Input: part model. Units: mm. Frame: model coordinates. A direction names the side the tool comes from. Round coordinates to 2 decimals unless told otherwise and drop trailing zeros. Loops run counter-clockwise (first coordinate to the right, second up) from the corner with the lowest first, then second, coordinate; pieces in that order, holes last.
1) Section B-B, the plane x = 12. Return loops of the section in (y, z).
2) First-contact query: pin 1 (0.8 mm diameter, centred on x = -17.5, y = 1, fed in from +Z); pin 2 (1.5 mm diameter, centred on x = 3.5, y = 30, fed in from +Z); pin 3 (1.5 mm diameter, centred on y = 35, z = 1.5, fed in from +X). Flat tips, straight axial feed; report the tip coordinate or a pass-through.
3) Section A-A, the plane z = 12.25. Return loops of the section in (x, y), and give its area (3 significant figures).
4) Section D-D, the plane x = -19. Return loops of the section in (y, z).
5) Access query for faces 5 (the face through (-17.5, 27, 2)), 6 (the face through (20, 22, 13)), 7 (the face through (-20, 41, 1)), 8 (the face through (-20, 10, 2)). Directions: +Z, -Z, +X, -X, +Y, -Y. A direction counts if a zero-diameter tool reaches every point of the face in a straight line with its end or side. Return the directions, or none.
6) Draft query along X for faces 1 (the face through (24.954, 22.465, 6.776)), 2 (the face through (-20.414, 22.465, 6.11)), 3 (the face through (-14.71, 55.68, 1.48)), 4 (the face through (18, 22, 16.75)). Return one class per face: pulls with the +X half, pulls with the -X half, needs draft (parallel to the pull), parting line crosses it, or undercut.
7) Ray query, line 1 along X through (y, z) = (56, 2.75); line 2 along Y through (x, z) = (-15, 2.1); line 3 along X through (y, z) = (21.5, 2). Return the intervals inside material, ascending.
8) Section C-C, the plane y = 11.5. Return loops of the section in (x, z).
from build123d import *

# Parameters (mm, degrees)
SKETCH1_W                 = 40
SKETCH1_H                 = 60
BOSS_EXTRUDE1_DEPTH       = 3
F_2_CLEARANCE_HOLE1_D     = 2.7051
F_2_CLEARANCE_HOLE1_DEPTH = 10
F_2_CLEARANCE_HOLE1_TIP   = 0.81269403
BOSS_EXTRUDE2_START       = -20
BOSS_EXTRUDE2_DEPTH       = 5
SKETCH6_R                 = 1.625
BOSS_EXTRUDE4_DEPTH       = 5
FILLET2_R                 = 0.25
SKETCH5_W                 = 5
SKETCH5_H                 = 2.5
BOSS_EXTRUDE3_DEPTH       = 3
BOSS_EXTRUDE5_DEPTH       = 3
F_4_CLEARANCE_HOLE1_D     = 3.2639
FILLET3_START             = -1
FILLET3_DEPTH             = 4
FILLET3_2_DEPTH           = 3


with BuildPart() as part:
    # Sketch1 → Boss-Extrude1 (new body)
    with BuildSketch(Plane.XY):
        with Locations((0, 30)):
            Rectangle(SKETCH1_W, SKETCH1_H)
        Polygon((-17.5, 54), (17.5, 54), (0, 30.744655424), align=None, mode=Mode.SUBTRACT)
        Polygon((-17.5, 49.010689152), (-17.5, 7.489310848), (-1.877266096, 28.25), align=None, mode=Mode.SUBTRACT)
        Polygon((17.5, 49.010689152), (1.877266096, 28.25), (17.5, 7.489310848), align=None, mode=Mode.SUBTRACT)
        Polygon((17.5, 2.5), (-17.5, 2.5), (0, 25.755344576), align=None, mode=Mode.SUBTRACT)
    extrude(amount=BOSS_EXTRUDE1_DEPTH)

    # #2 Clearance Hole1
    with Locations(Plane.XY.offset(3)):
        with Locations((-15, 57), (15, 57)):
            Hole(F_2_CLEARANCE_HOLE1_D / 2, depth=F_2_CLEARANCE_HOLE1_DEPTH)
            with Locations((0, 0, -(F_2_CLEARANCE_HOLE1_DEPTH + F_2_CLEARANCE_HOLE1_TIP / 2))):  # 118° drill point
                Cone(0, F_2_CLEARANCE_HOLE1_D / 2, F_2_CLEARANCE_HOLE1_TIP, mode=Mode.SUBTRACT)

    # Sketch4 → Boss-Extrude2 (add)
    with BuildSketch(Plane.XZ.offset(BOSS_EXTRUDE2_START)):
        Polygon((20, 3), (20, 16.75), (16, 16.75), (13.5, 14.25), (17.5, 14.25), (17.5, 3), align=None)
    boss_extrude2 = extrude(amount=-BOSS_EXTRUDE2_DEPTH)

    # Sketch6 → Boss-Extrude4 (add)
    with BuildSketch(Plane.XZ.offset(-20)):
        with BuildLine():
            Line((20, 8.882597042), (20, 0))
            Line((20, 0), (24.00871128, 3.363708157))
            ThreePointArc((24.00871128, 3.363708157), (24.93653944, 6.826409989), (22, 8.882597042))
            Line((22, 8.882597042), (20, 8.882597042))
        make_face()
        with Locations(Location((22, 5.757597042, 0), (0, 0, 270))):
            Circle(SKETCH6_R, mode=Mode.SUBTRACT)
    boss_extrude4 = extrude(amount=-BOSS_EXTRUDE4_DEPTH)

    # Mirror1: Boss-Extrude2, Boss-Extrude4 across plane
    add(boss_extrude2.mirror(Plane(origin=(0, 0, 0), x_dir=(0, 0, 1), z_dir=(1, 0, 0))))
    add(boss_extrude4.mirror(Plane(origin=(0, 0, 0), x_dir=(0, 0, 1), z_dir=(1, 0, 0))))

    # Fillet2
    fillet2_edges = [part.edges().sort_by_distance(p)[0] for p in [
        (-20, 22.5, 16.75),
        (-16, 22.5, 16.75),
        (-13.5, 22.5, 14.25),
        (-17.5, 22.5, 14.25),
        (17.5, 22.5, 14.25),
        (13.5, 22.5, 14.25),
        (16, 22.5, 16.75),
        (20, 22.5, 16.75),
    ]]
    fillet(fillet2_edges, radius=FILLET2_R)

    # Sketch5 → Boss-Extrude3 (add)
    with BuildSketch(Plane.XY.offset(3)):
        with Locations((17.5, 1.25)):
            Rectangle(SKETCH5_W, SKETCH5_H)
        with Locations((-17.5, 1.25)):
            Rectangle(SKETCH5_W, SKETCH5_H)
        with Locations((0, 55.25)):
            Rectangle(SKETCH5_W, SKETCH5_H)
    extrude(amount=BOSS_EXTRUDE3_DEPTH)

    # Sketch7 → Boss-Extrude5 (add)
    with BuildSketch(Plane(origin=(0, 0, 0), x_dir=(-1, 0, 0), z_dir=(0, 0, -1))):
        with BuildLine():
            Line((3.5, -3), (3.5, 0))
            Line((3.5, 0), (-3.5, 0))
            Line((-3.5, 0), (-3.5, -3))
            ThreePointArc((-3.5, -3), (0, -6.5), (3.5, -3))
        make_face()
    extrude(amount=-BOSS_EXTRUDE5_DEPTH)

    # #4 Clearance Hole1 (through all)
    with Locations(Plane.XY.offset(3)):
        with Locations((0, -3)):
            Hole(F_4_CLEARANCE_HOLE1_D / 2)

    # Fillet3: read off the stored shape, not the designer's step
    # Fillet3 outline → Fillet3 (cut)
    with BuildSketch(Plane.XY.offset(FILLET3_START)):
        with BuildLine():
            Line((-20, 60), (-20, 57))
            ThreePointArc((-20, 57), (-19.121320344, 59.121320344), (-17, 60))
            Line((-17, 60), (-20, 60))
        make_face()
        with BuildLine():
            Line((20, 60), (17, 60))
            ThreePointArc((17, 60), (19.121320344, 59.121320344), (20, 57))
            Line((20, 57), (20, 60))
        make_face()
    extrude(amount=FILLET3_DEPTH, mode=Mode.SUBTRACT)

    # Fillet3 2 outline → Fillet3 2 (add)
    with BuildSketch(Plane.XY):
        with BuildLine():
            Line((-3.5, 0), (-6.5, 0))
            ThreePointArc((-6.5, 0), (-4.378679656, -0.878679656), (-3.5, -3))
            Line((-3.5, -3), (-3.5, 0))
        make_face()
        with BuildLine():
            Line((3.5, 0), (3.5, -3))
            ThreePointArc((3.5, -3), (4.378679656, -0.878679656), (6.5, 0))
            Line((6.5, 0), (3.5, 0))
        make_face()
    extrude(amount=FILLET3_2_DEPTH)


solid = part.part
Final values:
1. outline: (0, 0) - (2.5, 0) - (2.5, 3) - (0, 3) - close; (9.81, 0) - (14.8, 0) - (14.8, 3) - (9.81, 3) - close; (41.7, 0) - (46.69, 0) - (46.69, 3) - (41.7, 3) - close; (54, 0) - (60, 0) - (60, 3) - (54, 3) - close
2. pin 1: stops at z = 6
2. pin 2: stops at z = 3
2. pin 3: stops at x = 20
3. outline: (-20, 20) - (-17.5, 20) - (-17.5, 25) - (-20, 25) - close; (17.5, 20) - (20, 20) - (20, 25) - (17.5, 25) - close
3. area: 25.0 mm2
4. outline: (0, 0) - (59.24, 0) - (59.24, 3) - (25, 3) - (25, 16.75) - (20, 16.75) - (20, 3) - (2.5, 3) - (2.5, 6) - (0, 6) - close
5. face 5: -Z
5. face 6: +Z, +X, +Y, -Y
5. face 7: +Z, -Z, -X, +Y
5. face 8: +Z, -Z, -X, -Y
6. face 1: pulls with the +X half
6. face 2: undercut
6. face 3: undercut
6. face 4: needs draft
7. line 1: x = -20 to -15.91, -14.09 to 14.09, 15.91 to 20
7. line 2: y = 0 to 2.5, 5.82 to 10.81, 45.69 to 50.68, 54 to 55.65, 58.35 to 60
7. line 3: x = -22.38 to -17.5, -6.96 to -3.2, 3.2 to 6.96, 17.5 to 22.38
8. outline: (-20, 0) - (-17.5, 0) - (-17.5, 3) - (-20, 3) - close; (-14.48, 0) - (-10.73, 0) - (-10.73, 3) - (-14.48, 3) - close; (10.73, 0) - (14.48, 0) - (14.48, 3) - (10.73, 3) - close; (17.5, 0) - (20, 0) - (20, 3) - (17.5, 3) - close
